Geometry check sheet. Reference: the model listing, model coordinates, mm. A direction names the side the tool comes from. Coordinates: 2 decimals unless noted, no trailing zeros. Loops run counter-clockwise (first coordinate to the right, second up) from the corner with the lowest first, then second, coordinate; pieces in that order, holes last. Notation, with made-up numbers: (61, 70) -> (109, 70) arc R19 ccw to (109, 84) -> close; hole circle Ø4 at (22.5, 4). An arc over 180 degrees is marked (long way). Answer as a JSON object with one key per item and string values.
from build123d import *

# Parameters (mm, degrees)
SKETCH1_W                                        = 365
SKETCH1_H                                        = 300
BOSS_EXTRUDE1_DEPTH                              = 30
SKETCH2_W                                        = 234
SKETCH2_H                                        = 300
SKETCH2_W_2                                      = 112.5
CUT_EXTRUDE1_DEPTH                               = 5
SKETCH3_W                                        = 305
SKETCH3_H                                        = 300
CUT_EXTRUDE2_DEPTH                               = 8
CBORE_FOR_M12_SOCKET_HEAD_CAP_SCREW1_D           = 14
CBORE_FOR_M12_SOCKET_HEAD_CAP_SCREW1_CBORE_D     = 20
CBORE_FOR_M12_SOCKET_HEAD_CAP_SCREW1_CBORE_DEPTH = 14
LPATTERN1_COUNT                                  = 2
LPATTERN1_PITCH                                  = 335
CBORE_FOR_M8_SOCKET_HEAD_CAP_SCREW1_D            = 9
CBORE_FOR_M8_SOCKET_HEAD_CAP_SCREW1_CBORE_D      = 14
CBORE_FOR_M8_SOCKET_HEAD_CAP_SCREW1_CBORE_DEPTH  = 9
LPATTERN2_COUNT                                  = 2
LPATTERN2_PITCH                                  = 210
LPATTERN2_COUNT_DIR2                             = 2
LPATTERN2_PITCH_DIR2                             = 168
CBORE_FOR_M10_SOCKET_HEAD_CAP_SCREW1_D           = 12
CBORE_FOR_M10_SOCKET_HEAD_CAP_SCREW1_CBORE_D     = 18
CBORE_FOR_M10_SOCKET_HEAD_CAP_SCREW1_CBORE_DEPTH = 11


with BuildPart() as part:
    # Sketch1 → Boss-Extrude1 (new body)
    with BuildSketch(Plane.XY):
        with Locations((-182.5, 150)):
            Rectangle(SKETCH1_W, SKETCH1_H)
    extrude(amount=-BOSS_EXTRUDE1_DEPTH)

    # Sketch2 → Cut-Extrude1 (cut)
    with BuildSketch(Plane(origin=(0, 0, -30), x_dir=(-1, 0, 0), z_dir=(0, 0, -1))):
        with Locations((117, 150)):
            Rectangle(SKETCH2_W, SKETCH2_H)
        with Locations((308.75, 150)):
            Rectangle(SKETCH2_W_2, SKETCH2_H)
    extrude(amount=-CUT_EXTRUDE1_DEPTH, mode=Mode.SUBTRACT)

    # Sketch3 → Cut-Extrude2 (cut)
    with BuildSketch(Plane.XY):
        with Locations((-182.5, 150)):
            Rectangle(SKETCH3_W, SKETCH3_H)
    extrude(amount=-CUT_EXTRUDE2_DEPTH, mode=Mode.SUBTRACT)

    # CBORE for M12 Socket Head Cap Screw1 (through all)
    with Locations(Plane(origin=(-5.933420532, 68.021379898, -25), x_dir=(1, 0, 0), z_dir=(0, 0, -1))):
        with Locations((-9.066579468, -201.978620102), (-9.066579468, -129.978620102), (-9.066579468, -33.978620102), (-9.066579468, 38.021379898)):
            cbore_for_m12_socket_head_cap_screw1 = CounterBoreHole(CBORE_FOR_M12_SOCKET_HEAD_CAP_SCREW1_D / 2, CBORE_FOR_M12_SOCKET_HEAD_CAP_SCREW1_CBORE_D / 2, CBORE_FOR_M12_SOCKET_HEAD_CAP_SCREW1_CBORE_DEPTH)

    # LPattern1: CBORE for M12 Socket Head Cap Screw1 ×2
    with Locations(*[(-i * LPATTERN1_PITCH, 0, 0) for i in range(1, LPATTERN1_COUNT)]):
        add(cbore_for_m12_socket_head_cap_screw1, mode=Mode.SUBTRACT)

    # CBORE for M8 Socket Head Cap Screw1 (through all)
    with Locations(Plane.XY.offset(-8)):
        with Locations((-52.5, 30), (-52.5, 102), (-102.5, 102), (-102.5, 30)):
            cbore_for_m8_socket_head_cap_screw1 = CounterBoreHole(CBORE_FOR_M8_SOCKET_HEAD_CAP_SCREW1_D / 2, CBORE_FOR_M8_SOCKET_HEAD_CAP_SCREW1_CBORE_D / 2, CBORE_FOR_M8_SOCKET_HEAD_CAP_SCREW1_CBORE_DEPTH)

    # LPattern2: CBORE for M8 Socket Head Cap Screw1 2 × 2
    with Locations(*[(-i * LPATTERN2_PITCH, j * LPATTERN2_PITCH_DIR2, 0) for i in range(LPATTERN2_COUNT) for j in range(LPATTERN2_COUNT_DIR2) if (i, j) != (0, 0)]):
        add(cbore_for_m8_socket_head_cap_screw1, mode=Mode.SUBTRACT)

    # CBORE for M10 Socket Head Cap Screw1 (through all)
    with Locations(Plane.XY.offset(-8)):
        with Locations((-152.5, 240), (-152.5, 180), (-212.5, 180), (-212.5, 240)):
            CounterBoreHole(CBORE_FOR_M10_SOCKET_HEAD_CAP_SCREW1_D / 2, CBORE_FOR_M10_SOCKET_HEAD_CAP_SCREW1_CBORE_D / 2, CBORE_FOR_M10_SOCKET_HEAD_CAP_SCREW1_CBORE_DEPTH)


solid = part.part
1. Thickness scan on probe 1 along Y at (x, z) = (-262.5, -18.75); probe 2 along Y at (x, z) = (-212.5, -16); probe 3 along Y at (x, z) = (-16, -23.5). Record the ranges inside material, lowest first. Write a range as from..to.
Evaluation:
{"probe 1": "y = 0..25.5, 34.5..97.5, 106.5..193.5, 202.5..265.5, 274.5..300", "probe 2": "y = 0..171, 189..231, 249..300", "probe 3": "y = 0..20.05, 39.95..92.05, 111.95..188.05, 207.95..260.05, 279.95..300"}
2. Section check D-D, the plane x = -243. Record the boundary of the cut face in (y, z).
Evaluation:
{"outline": "(0, -30) -> (300, -30) -> (300, -8) -> (0, -8) -> close"}
3. Tool access check on faces 1 (the face through (-208.08, 244.06, -22.04)), 2 (the face through (-10.386, 278.872, -18.098)), 3 (the face through (-103, 265, -17)). Record the directions out of +Z, -Z, +X, -X, +Y, -Y that give a thin tool (end or side, any length) a straight path to the whole face; none if there is none.
Evaluation:
{"face 1": "+Z, -Z", "face 2": "-Z", "face 3": "+Z"}
4. Section check A-A, the plane y = 128. Record the boundary of the cut face in (x, z).
Evaluation:
{"outline": "(-365, -25) -> (-252.5, -25) -> (-252.5, -30) -> (-234, -30) -> (-234, -25) -> (0, -25) -> (0, 0) -> (-30, 0) -> (-30, -8) -> (-335, -8) -> (-335, 0) -> (-365, 0) -> close"}
5. Section check B-B, the plane x = -15. State how many separate pieces and enclosed holes the cut face has, then the cut area to 3 significant figures.
Evaluation:
{"separate pieces": "5", "enclosed holes": "0", "area": "5,760 mm^2"}
6. Depth check by flat-ended pin: P1, Ø5.5, axis at x = -102.5, y = 30, coming from the -Z side; P2, Ø11.5, axis at x = -312.5, y = 198, coming from the -Z side; P3, Ø20, axis at x = -214.5, y = 244, coming from the +Z side; P4, Ø18, axis at x = -350, y = 198, coming from the -Z side. Enter the tip coordinate at first touch or a pass-through.
Evaluation:
{"P1": "passes through", "P2": "stops at z = -25", "P3": "stops at z = -8", "P4": "stops at z = -11"}
7. Mould release check, pull along Y, two halves, no side actions. Record for faces 4 (the face through (-104.017, 263.166, -12.437)), 5 (the face through (-335, 148, -4)), 6 (the face through (-185, 300, -15)): released by +Y, released by -Y, zero draft, split by the parting line, or undercut.
Evaluation:
{"face 4": "undercut", "face 5": "zero draft", "face 6": "released by +Y"}
